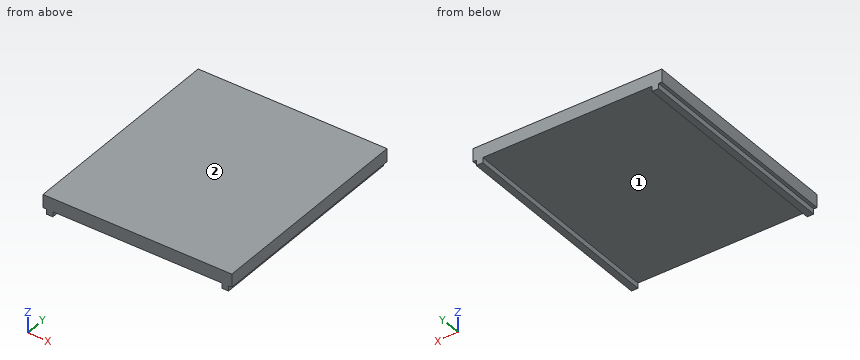
```python
from build123d import *

# Parameters (mm, degrees)
SKETCH3_W           = 29
SKETCH3_H           = 33
BOSS_EXTRUDE1_DEPTH = 2
SKETCH5_W           = 1
SKETCH5_H           = 33
BOSS_EXTRUDE2_DEPTH = 0.8


with BuildPart() as part:
    # Sketch3 → Boss-Extrude1 (new body)
    with BuildSketch(Plane.XY.offset(1)):
        Rectangle(SKETCH3_W, SKETCH3_H)
    extrude(amount=BOSS_EXTRUDE1_DEPTH)

    # Sketch5 → Boss-Extrude2 (add)
    with BuildSketch(Plane(origin=(0, 0, 1), x_dir=(-1, 0, 0), z_dir=(0, 0, -1))):
        with Locations((13.5, 0)):
            Rectangle(SKETCH5_W, SKETCH5_H)
        with Locations((-13.5, 0)):
            Rectangle(SKETCH5_W, SKETCH5_H)
    extrude(amount=BOSS_EXTRUDE2_DEPTH)


solid = part.part
```
Source: CAD feature listing. Evaluate the final solid. Frame: model axes, mm. Face numbers are marked on the shaded views. Round coordinates to 2 decimals unless told otherwise and drop trailing zeros. Loops run counter-clockwise (first coordinate to the right, second up) from the corner with the lowest first, then second, coordinate; pieces in that order, holes last. Notation, with made-up numbers: M 72.5,-10.75 L 93.5,-10.75 A26 cw 93.5,10.25 Z; hole C 50.5,-26.75 d8. An arc over 180 degrees is marked long. Use a Markdown table: item, result. Add a question column.
1. Section query B-B on x = -3. Return the cut outline in (y, z).
2. Section query A-A on y = 7. Return the cut outline in (x, z).
3. Contact query for flat-ended pins moving along their axis: P1, Ø0.9, axis at y = -2.5, z = 0.5, coming from the -X side; P2, Ø0.6, axis at y = 8, z = 0.5, coming from the +X side; P3, Ø1, axis at x = -8, y = 8.5, coming from the -Z side. Output: stop coordinate, or through.
4. Line query: line 1 (X direction, y = -11, z = 0.7); line 2 (Z direction, x = 6.75, y = 3.5). Output: solid intervals per line, ascending.
5. Mould query, pull axis X, two halves, no side actions, for the marked faces 1 and 2. Classes: pulls with the +X half, pulls with the -X half, needs draft (parallel to the pull), parting line crosses it, or undercut.
Reported:
| question | item | result |
|---|---|---|
| 1 | outline | M -16.5,1 L 16.5,1 L 16.5,3 L -16.5,3 Z |
| 2 | outline | M -14.5,1 L -14,1 L -14,0.2 L -13,0.2 L -13,1 L 13,1 L 13,0.2 L 14,0.2 L 14,1 L 14.5,1 L 14.5,3 L -14.5,3 Z |
| 3 | P1 | stops at x = -14 |
| 3 | P2 | stops at x = 14 |
| 3 | P3 | stops at z = 1 |
| 4 | line 1 | x = -14 to -13, 13 to 14 |
| 4 | line 2 | z = 1 to 3 |
| 5 | face 1 | undercut |
| 5 | face 2 | needs draft |
